Geometry check sheet. Reference: the model listing, model coordinates, mm. Coordinates: 2 decimals unless noted, no trailing zeros. Order: outer loops, then holes, each group sorted by start corner. A loop starts at its lowest first (then second) coordinate and runs counter-clockwise, first axis right, second up. Notation, with made-up numbers: (-35, 49.25) -> (11, 49.25) arc R36 ccw to (11, 86.25) -> close; hole circle Ø9 at (-24, 67.5). An arc over 180 degrees is marked (long way). Answer in a Markdown table with one row per item. Add a question column.
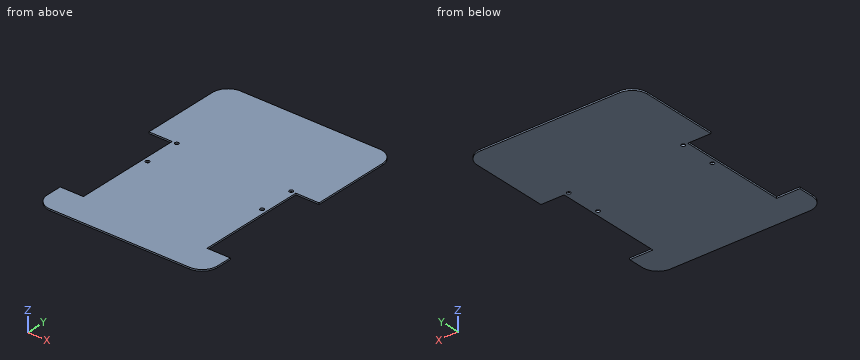
```python
from build123d import *

# Parameters (mm, degrees)
F1_DEPTH = 1
F3_D     = 2.5


# Not quite as in the source:
# - a feature names something its author has since deleted; it is built from what else it names


with BuildPart() as f1:
    # F0 (on Top) → F1 (new body)
    with BuildSketch(Plane.XY):
        with BuildLine():
            Line((45, 0), (-45, 0))
            ThreePointArc((-45, 0), (-52.0710678119, -2.9289321881), (-55, -10))
            Line((-55, -10), (-55, -60))
            Line((-55, -60), (-40, -60))
            Line((-40, -60), (-40, -130))
            Line((-40, -130), (-55, -130))
            Line((-55, -130), (-55, -140))
            ThreePointArc((-55, -140), (-52.0710678119, -147.0710678119), (-45, -150))
            Line((-45, -150), (45, -150))
            ThreePointArc((45, -150), (52.0710678119, -147.0710678119), (55, -140))
            Line((55, -140), (55, -130))
            Line((55, -130), (40, -130))
            Line((40, -130), (40, -60))
            Line((40, -60), (55, -60))
            Line((55, -60), (55, -10))
            ThreePointArc((55, -10), (52.0710678119, -2.9289321881), (45, 0))
        make_face()
    extrude(amount=F1_DEPTH)

    # F3 (through all)
    with Locations(Plane.XY.offset(1)):
        with Locations((37, -60), (37, -83), (-37, -60), (-37, -83)):
            Hole(F3_D / 2)


solid = f1.part
```
(1) Cross-section at B-B (y = -123). Enter the section's corners in (x, z), plus the area to 3 significant figures.
(2) Go/stop test with a flat-tipped pin: P1, Ø1.5, axis at x = -37, y = -60, coming from the -Z side. Record where the tip stops, or that it passes through.
(3) Cross-section at A-A (z = 0.55). Enter the section's corners in (x, y), plus the area to 3 significant figures.
(4) Scan lines: line 1 along Y through (x, z) = (37, 0.7); line 2 along X through (y, z) = (-83, 0.4); line 3 along Y through (x, z) = (-42.5, 0.25). Record each from-to range of solid material in increasing order.
Checks:
| question | item | result |
|---|---|---|
| 1 | outline | (-40, 0) -> (40, 0) -> (40, 1) -> (-40, 1) -> close |
| 1 | area | 80.0 mm² |
| 2 | P1 | through |
| 3 | outline | (-55, -140) arc R10 ccw to (-45, -150) -> (45, -150) arc R10 ccw to (55, -140) -> (55, -130) -> (40, -130) -> (40, -60) -> (55, -60) -> (55, -10) arc R10 ccw to (45, 0) -> (-45, 0) arc R10 ccw to (-55, -10) -> (-55, -60) -> (-40, -60) -> (-40, -130) -> (-55, -130) -> close; hole circle Ø2.5 at (-37, -83); hole circle Ø2.5 at (-37, -60); hole circle Ø2.5 at (37, -83); hole circle Ø2.5 at (37, -60) |
| 3 | area | 14,300 mm² |
| 4 | line 1 | -150 to -84.25, -81.75 to -61.25, -58.75 to 0 |
| 4 | line 2 | -40 to -38.25, -35.75 to 35.75, 38.25 to 40 |
| 4 | line 3 | -150 to -130, -60 to 0 |
